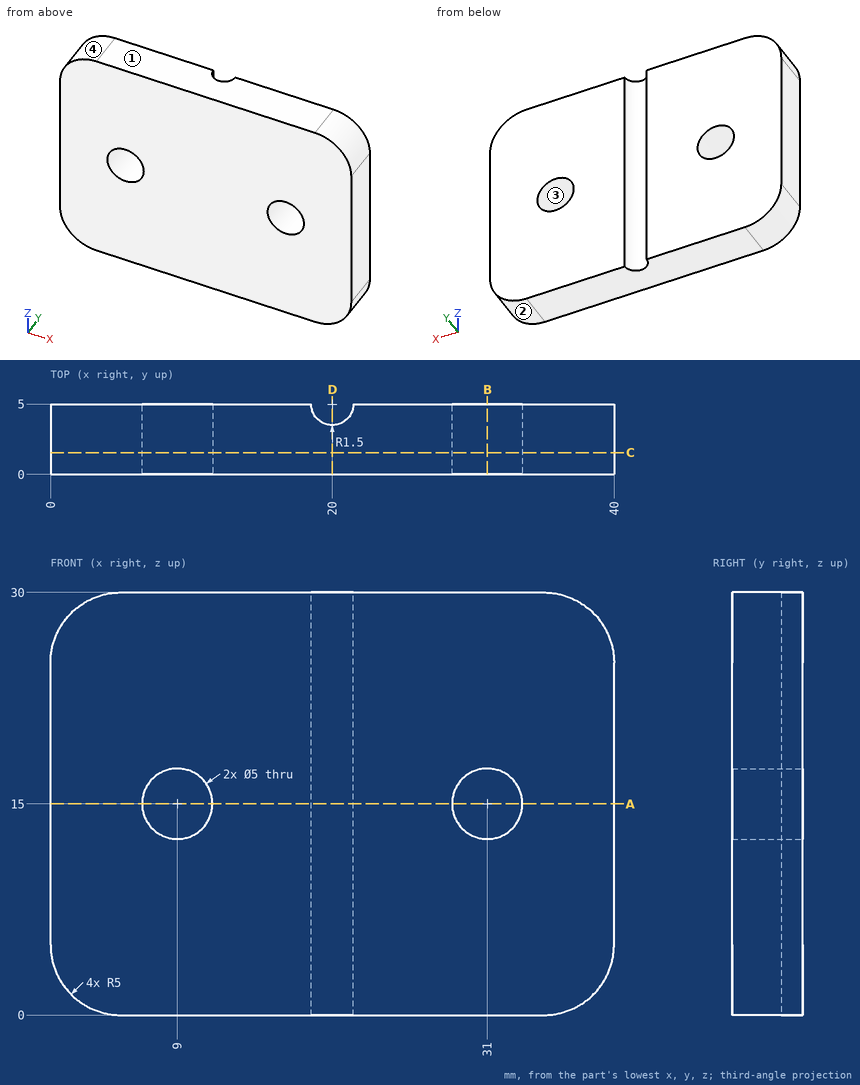
Design review of the part shown in the three views and the two pictorial views. Dimensions are in mm from the part's minimum x, y and z. Coordinates: 2 decimals unless noted, no trailing zeros. Loops run counter-clockwise (first coordinate to the right, second up) from the corner with the lowest first, then second, coordinate; pieces in that order, holes last. Notation, with made-up numbers: (26.5, -37) - (30.5, -37) arc R7 ccw to (30.5, -24) - close; hole circle Ø8 at (-6, -32). An arc over 180 degrees is marked (long way). Use a Markdown table: item, result. Add a question column.
Item 1: We need section B-B (x = 31). Give the boundary of the cut face in (y, z).
Item 2: Insertion check: pin 1 Ø1.5 at (y, z) = (3, 15) entering from -X; pin 2 Ø3 at (x, z) = (31, 15) entering from -Y. Each pin has a flat end and moves straight along its axis. Give the tip position at first contact, or say it passes through.
Item 3: We need section A-A (z = 15). Give the boundary of the cut face in (x, y).
Item 4: For line 1 (Z direction, x = 31, y = 2.1); line 2 (X direction, y = 4.55, z = 15.75); line 3 (Z direction, x = 11, y = 1.95), list the stretches that pass through material, from the lowest coordinate up.
Item 5: We need section C-C (y = 1.55). Give the boundary of the cut face in (x, z), and give its area (3 significant figures).
Item 6: We need section D-D (x = 20). Give the boundary of the cut face in (y, z), and give its area (3 significant figures).
Item 7: Mouldability with a two-part tool opening along X and no side actions: class the marked faces 1, 2, 3 and 4 as pulls with the +X half, pulls with the -X half, needs draft (parallel to the pull), parting line crosses it, or undercut.
Results list:
| question | item | result |
|---|---|---|
| 1 | outline | (0, 0) - (5, 0) - (5, 12.5) - (0, 12.5) - close; (0, 17.5) - (5, 17.5) - (5, 30) - (0, 30) - close |
| 2 | pin 1 | stops at x = 0 |
| 2 | pin 2 | passes through |
| 3 | outline | (0, 0) - (6.5, 0) - (6.5, 5) - (0, 5) - close; (11.5, 0) - (28.5, 0) - (28.5, 5) - (21.5, 5) arc R1.5 cw to (18.5, 5) - (11.5, 5) - close; (33.5, 0) - (40, 0) - (40, 5) - (33.5, 5) - close |
| 4 | line 1 | z = 0 to 12.5, 17.5 to 30 |
| 4 | line 2 | x = 0 to 6.62, 11.38 to 18.57, 21.43 to 28.62, 33.38 to 40 |
| 4 | line 3 | z = 0 to 13.5, 16.5 to 30 |
| 5 | outline | (0, 5) arc R5 ccw to (5, 0) - (35, 0) arc R5 ccw to (40, 5) - (40, 25) arc R5 ccw to (35, 30) - (5, 30) arc R5 ccw to (0, 25) - close; hole circle Ø5 at (9, 15); hole circle Ø5 at (31, 15) |
| 5 | area | 1,140 mm^2 |
| 6 | outline | (0, 0) - (3.5, 0) - (3.5, 30) - (0, 30) - close |
| 6 | area | 105 mm^2 |
| 7 | face 1 | needs draft |
| 7 | face 2 | pulls with the +X half |
| 7 | face 3 | undercut |
| 7 | face 4 | pulls with the -X half |
